The model under review builds one solid part; all positions refer to its coordinate system, in mm. Coordinates: 2 decimals unless noted, no trailing zeros. Order: outer loops, then holes, each group sorted by start corner. A loop starts at its lowest first (then second) coordinate and runs counter-clockwise, first axis right, second up. Notation, with made-up numbers: (87.25, 5) -> (96.25, 5) arc R21 ccw to (96.25, 33) -> close; hole circle Ø2 at (20.25, 83.5). An arc over 180 degrees is marked (long way). Put each result on its own line as item: value.
from build123d import *

# Parameters (mm, degrees)
SKETCH1_R           = 3
SKETCH1_R_2         = 1.5
BOSS_EXTRUDE1_DEPTH = 1.5
FILLET1_R           = 7


with BuildPart() as part:
    # Sketch1 → Boss-Extrude1 (new, symmetric)
    with BuildSketch(Plane(origin=(0, 0, 0), x_dir=(1, 0, 0), z_dir=(0, 1, 0))):
        with BuildLine():
            Line((-4.497129186, 14.160714286), (-4.996810207, 0.178571429))
            ThreePointArc((-4.996810207, 0.178571429), (-3.340250682, -3.720581323), (0.714285714, -4.948716593))
            Line((0.714285714, -4.948716593), (14.428571429, -2.969229956))
            ThreePointArc((14.428571429, -2.969229956), (17, 0), (14.428571429, 2.969229956))
            Line((14.428571429, 2.969229956), (4.847659913, 4.352115416))
            Line((4.847659913, 4.352115416), (4.497129186, 14.160714286))
            ThreePointArc((4.497129186, 14.160714286), (0, 18.5), (-4.497129186, 14.160714286))
        make_face()
        with Locations(Location((0, 0, 0), (0, 0, 270))):
            Circle(SKETCH1_R, mode=Mode.SUBTRACT)
        with Locations(Location((14, 0, 0), (0, 0, 270))):
            Circle(SKETCH1_R_2, mode=Mode.SUBTRACT)
    extrude(amount=BOSS_EXTRUDE1_DEPTH, both=True)

    # Cut-Loft1: read off the stored shape, not the designer's step
    # Cut-Loft1: loft between two sections, ruled curve by curve
    cut_loft1_from = [
        Edge.make_bspline([(-3.051453725, 1.5, -15.949985604), (0.848517484, 1.5, -22.052893053), (6.951424933, 1.5, -18.152921845), (3.051453725, 1.5, -12.050014396), (-0.848517484, 1.5, -5.947106947), (-6.951424933, 1.5, -9.847078155), (-3.051453725, 1.5, -15.949985604)], [0, 0, 0, 0, 0.5, 0.5, 0.5, 1, 1, 1, 1], 3, [1, 0.333333333, 0.333333333, 1, 0.333333333, 0.333333333, 1]),
    ]
    cut_loft1_to = [
        Edge.make_bspline([(-1.172439921, 0, -15.767875328), (2.363310734, 0, -18.11275517), (4.708190576, 0, -14.577004515), (1.172439921, 0, -12.232124672), (-2.363310734, 0, -9.88724483), (-4.708190576, 0, -13.422995485), (-1.172439921, 0, -15.767875328)], [0, 0, 0, 0, 0.5, 0.5, 0.5, 1, 1, 1, 1], 3, [1, 0.333333333, 0.333333333, 1, 0.333333333, 0.333333333, 1]),
    ]
    cut_loft1 = Solid(Shell([*[Face.make_surface_from_curves(cut_loft1_from[k], cut_loft1_to[k]) for k in range(1)], Face(Wire(cut_loft1_from)), Face(Wire(cut_loft1_to))]))
    add(cut_loft1, mode=Mode.SUBTRACT)

    # Fillet1
    fillet1_edges = [part.edges().sort_by_distance(p)[0] for p in [
        (4.847659913, 0, -4.352115416),
    ]]
    fillet(fillet1_edges, radius=FILLET1_R)

    # Mirror1: Cut-Loft1 across plane
    add(cut_loft1.mirror(Plane.ZX), mode=Mode.SUBTRACT)


solid = part.part
Item 1: Consider section D-D on x = 8.5. Write out the cut boundary in (y, z), and give its area (3 significant figures).
Answers below:
outline: (-1.5, -4.19) -> (1.5, -4.19) -> (1.5, 3.82) -> (-1.5, 3.82) -> close
area: 24.0 mm^2
Item 2: Consider section A-A on x = 14. Write out the cut boundary in (y, z), and give its area (3 significant figures).
Answers below:
outline: (-1.5, -3.03) -> (1.5, -3.03) -> (1.5, -1.5) -> (-1.5, -1.5) -> close; (-1.5, 1.5) -> (1.5, 1.5) -> (1.5, 3.03) -> (-1.5, 3.03) -> close
area: 9.19 mm^2
Item 3: Mouldability with a two-part tool opening along Z and no side actions: class faces 1 (the cylindrical face through (0.1, 0, -18.5)), 2 (the cylindrical face through (14.45, -0.02, 1.43)), 3 (the cylindrical face through (17, 0, 0)), 4 (the cylindrical face through (0.9, -0.02, 2.86)) as +Z half, -Z half, draft (parallel to the pull), parting line (faces both ways), or undercut.
Answers below:
face 1: -Z half
face 2: undercut
face 3: parting line
face 4: undercut
Item 4: For line 1 (X direction, y = -0.4, z = 0); line 2 (X direction, y = 0.2, z = -1); line 3 (Z direction, x = -2, y = -1.2), list the stretches that pass through material, from the lowest coordinate up. Write a range as from..to.
Answers below:
line 1: -5..-3, 3..12.5, 15.5..17
line 2: -4.97..-2.83, 2.83..12.88, 15.12..16.83
line 3: -18.03..-16.61, -11.39..-2.24, 2.24..4.58
Item 5: For pin 1 Ø5 at (x, z) = (0, 0) entering from +Y; pin 2 Ø1.5 at (y, z) = (0, -8) entering from -X; pin 3 Ø1 at (y, z) = (-0.5, -5) entering from +X, all flat-tipped, find the tip position at first contact; note any pin that passes through.
Answers below:
pin 1: through
pin 2: x = -4.74
pin 3: x = 7.94
Item 6: Consider section B-B on x = 0. Count the separate pieces of the cut face and the enclosed holes in it, and give its area (3 significant figures).
Answers below:
separate pieces: 3
enclosed holes: 0
area: 35.5 mm^2
